Geometry check sheet. Reference: the model listing, model coordinates, mm. Face numbers are marked on the shaded views. A direction names the side the tool comes from. Round coordinates to 2 decimals unless told otherwise and drop trailing zeros. Write each loop counter-clockwise with the first axis right and the second up, starting at its lowest first coordinate (ties: lowest second). Pieces come first, ordered by that corner, then holes. Notation, with made-up numbers: (84, -34) -> (131, -34) arc R15 cw to (131, -14) -> close; hole circle Ø1 at (84, 81.5). An arc over 180 degrees is marked (long way). Return JSON: item names as keys, results as strings. Group by question number.
from build123d import *


with BuildPart() as part:
    # Sketch1 → Revolve1 (revolve)
    with BuildSketch(Plane(origin=(0, 0, 0), x_dir=(0, 0, -1), z_dir=(1, 0, 0)), mode=Mode.PRIVATE) as revolve1_sk:
        Polygon((-142.749573327, 73.502909781), (-92.749573327, 73.502909781), (-92.749573327, 50.502909781), (-94.749573327, 50.502909781), (-94.749573327, 52.502909781), (-95.749573327, 52.502909781), (-95.749573327, 50.502909781), (-97.749573327, 50.502909781), (-97.749573327, 52.502909781), (-98.749573327, 52.502909781), (-98.749573327, 50.502909781), (-107.749573327, 50.502909781), (-107.749573327, 51.502909781), (-108.749573327, 51.502909781), (-108.749573327, 48.502909781), (-126.749573327, 48.502909781), (-126.749573327, 51.502909781), (-127.749573327, 51.502909781), (-127.749573327, 50.502909781), (-136.749573327, 50.502909781), (-136.749573327, 52.502909781), (-137.749573327, 52.502909781), (-137.749573327, 50.502909781), (-139.749573327, 50.502909781), (-139.749573327, 52.502909781), (-140.749573327, 52.502909781), (-140.749573327, 50.502909781), (-142.749573327, 50.502909781), align=None)
    revolve(revolve1_sk.sketch.rotate(Axis((0, -1.497090219, 168.192153132), (0, 0, -1)), 90), axis=Axis((0, -1.497090219, 168.192153132), (0, 0, -1)))


solid = part.part
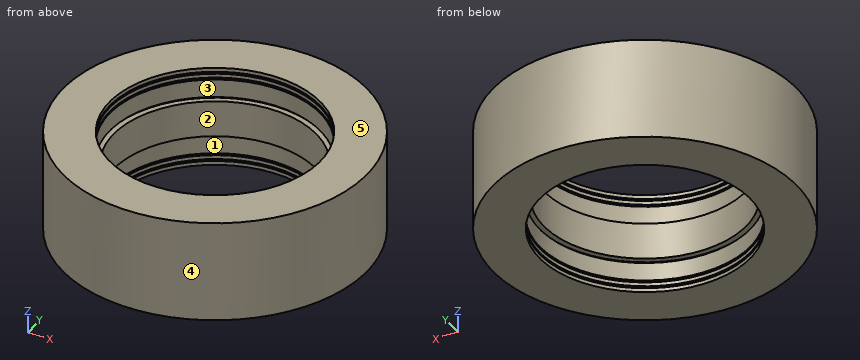
1) Sectioned sample at C-C on x = -58. Enter the section's corners in (y, z), and give its area (4 significant figures).
2) Go/stop test with flat-tipped pins: P1, Ø12, axis at x = 4, z = 132.5, coming from the +Y side; P2, Ø12, axis at y = -33.5, z = 117.5, coming from the +X side; P3, Ø5, axis at y = 34.5, z = 134, coming from the -X side. Record where each tip stops, or that it passes through.
3) Tool access check on the marked faces 1 and 2. Record the directions out of +Z, -Z, +X, -X, +Y, -Y that give a thin tool (end or side, any length) a straight path to the whole face; none if there is none.
4) Material ranges on probe 1 along Y at (x, z) = (0, 117); probe 2 along Y at (x, z) = (0, 140); probe 3 along X at (y, z) = (24, 96.5), recorded low to high. Write a range as [from, to].
5) Sectioned sample at B-B on y = 58.5. Enter the section's corners in (x, z), and give its area (3 significant figures).
6) Sectioned sample at A-A on z = 104. Enter the section's corners in (x, y).
7) Sectioned sample at D-D on z = 112.5. Enter the section's corners in (x, y), and give its area (3 significant figures).
8) Mould release check, pull along X, two halves, no side actions. Record for the marked faces 3, 4 and 5: +X half, -X half, draft (parallel to the pull), parting line (faces both ways), or undercut.
Evaluation:
{
 "1": {"outline": "(-49.05, 92.75) -> (46.05, 92.75) -> (46.05, 142.75) -> (-49.05, 142.75) -> close", "area": "4,755 mm2"},
 "2": {"P1": "stops at y = 73.5", "P2": "stops at x = 70.35", "P3": "stops at x = -67.1"},
 "3": {"face 1": "-Z", "face 2": "+Z, -Z"},
 "4": {"probe 1": "y = [-76.5, -51.5], [48.5, 73.5]", "probe 2": "y = [-76.5, -55.5], [52.5, 73.5]", "probe 3": "x = [-70.53, -45.32], [45.32, 70.53]"},
 "5": {"outline": "(-45, 92.75) -> (45, 92.75) -> (45, 142.75) -> (-45, 142.75) -> close", "area": "4,500 mm2"},
 "6": {"outline": "circle Ø150 at (0, -1.5); hole circle Ø104 at (0, -1.5)"},
 "7": {"outline": "circle Ø150 at (0, -1.5); hole circle Ø100 at (0, -1.5)", "area": "9,820 mm2"},
 "8": {"face 3": "undercut", "face 4": "parting line", "face 5": "draft"}
}
